```python
from build123d import *

# Parameters (mm, degrees)
SKETCH1_W           = 22.098
SKETCH1_H           = 19.05
BOSS_EXTRUDE1_DEPTH = 23.749
SKETCH2_R           = 2.5527
CUT_EXTRUDE1_DEPTH  = 38.619663808
SHELL1_T            = -1.000000032


with BuildPart() as part:
    # Sketch1 → Boss-Extrude1 (new, symmetric)
    with BuildSketch(Plane(origin=(0, 0, 0), x_dir=(1, 0, 0), z_dir=(0, 1, 0))):
        with Locations((11.049, 9.525)):
            Rectangle(SKETCH1_W, SKETCH1_H)
    extrude(amount=BOSS_EXTRUDE1_DEPTH, both=True)

    # Sketch2 → Cut-Extrude1 (cut, through all)
    with BuildSketch(Plane.ZY):
        with Locations((-12.7, 12.7635)):
            Circle(SKETCH2_R)
        with Locations((-12.7, -12.6365)):
            Circle(SKETCH2_R)
        with Locations((-12.7, 0.0635)):
            Circle(SKETCH2_R)
    extrude(amount=-CUT_EXTRUDE1_DEPTH, mode=Mode.SUBTRACT)

    # Shell1
    shell1_openings = [part.faces().sort_by_distance(p)[0] for p in [
        (11.049, 12.7635, -15.2527),
        (11.049, -12.6365, -15.2527),
        (11.049, 0.0635, -15.2527),
        (11.049, 0, -19.05),
        (11.049, 0, 0),
    ]]
    offset(amount=SHELL1_T, openings=shell1_openings, kind=Kind.INTERSECTION)


solid = part.part
```
Can you work these out from the model? Positions are in its coordinate system, mm. A direction names the side the tool comes from. Coordinates: 2 decimals unless noted, no trailing zeros. Write each loop counter-clockwise with the first axis right and the second up, starting at its lowest first coordinate (ties: lowest second). Pieces come first, ordered by that corner, then holes. Notation, with made-up numbers: M -30.75,83.5 L 3.25,83.5 A19 cw 3.25,109.5 Z; hole C -18,-26 d6. An arc over 180 degrees is marked long. Write item = value, one per line. Start each with the question number.
Q1. Thinking about a two-plate mould opening in Z: for faces 3 (the face through (0.4, 0.1, -19.05)), 4 (the face through (21.591, -11.87, -10.265)), 5 (the face through (21.098, 0, -9)), which applies, released by +Z, released by -Z, zero draft, split by the parting line, or undercut?
Q2. If I drill on L1, parallel to Y at x = 21.8, z = -12.7; L2, parallel to X at y = -8.5, z = -13.25; L3, parallel to Y at x = 17.75, z = -1.25, over which ranges is the centre line in solid material (lowest first)? Write a range as [from, to].
Q3. On a 3-axis mill with a long thin cutter (end or side, diameter ignored), from which of +Z, -Z, +X, -X, +Y, -Y can I reach the whole of each face in a straight line? I mean faces 1 (the face through (1, 0, -9)), 2 (the face through (0.49, -0.91, -10.34)). Say none if no direction works.
Q4. I'm going to push a flat-ended pin straight in: pin 1 (6.5 mm diameter, centred on y = 0.06, z = -12.7, fed in from -X). Where does the tip first touch, or does it pass through?
Q5. If we section it at D-D, the plane y = -0.5: Write out the boundary of the cut face in (x, z), then the cut area to 3 significant figures.
Q6. If we section it at C-C, the plane z = -12.7: State how many separate pieces and enclosed holes the cut face has, then the cut area to 3 significant figures.
Q7. If we section it at A-A, the plane x = 16.75: Write out the boundary of the cut face in (y, z), then the cut area to 3 significant figures.
Q8. If we section it at B-B, the plane y = 8: Write out the boundary of the cut face in (x, z).
Check sheet entries:
q1.face_3 = released by -Z
q1.face_4 = undercut
q1.face_5 = zero draft
q2.L1 = [-23.75, -15.19], [-10.08, -2.49], [2.62, 10.21], [15.32, 23.75]
q2.L2 = [0, 1], [21.1, 22.1]
q2.L3 = [-23.75, -22.75], [22.75, 23.75]
q3.face_1 = +Z, -Z
q3.face_2 = +X, -X
q4.pin_1 = 0
q5.outline = M 0,-19.05 L 1,-19.05 L 1,-15.19 L 0,-15.19 Z; M 0,-10.21 L 1,-10.21 L 1,0 L 0,0 Z; M 21.1,-19.05 L 22.1,-19.05 L 22.1,-15.19 L 21.1,-15.19 Z; M 21.1,-10.21 L 22.1,-10.21 L 22.1,0 L 21.1,0 Z
q5.area = 28.1 mm²
q6.separate_pieces = 6
q6.enclosed_holes = 0
q6.area = 105 mm²
q7.outline = M -23.75,-19.05 L -22.75,-19.05 L -22.75,0 L -23.75,0 Z; M 22.75,-19.05 L 23.75,-19.05 L 23.75,0 L 22.75,0 Z
q7.area = 38.1 mm²
q8.outline = M 0,-19.05 L 1,-19.05 L 1,0 L 0,0 Z; M 21.1,-19.05 L 22.1,-19.05 L 22.1,0 L 21.1,0 Z
